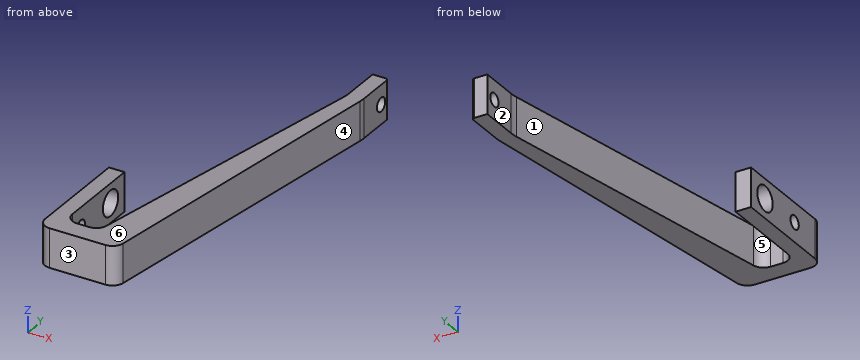
```python
from build123d import *

# Parameters (mm, degrees)
F0_W     = 4
F0_H     = 25
F1_DEPTH = 10
F2_R     = 3
F3_R     = 10
F4_R     = 1.75
F5_DEPTH = 5
F6_R     = 3.25
F6_R_2   = 1.75
F7_DEPTH = 6
F8_R     = 0.7


# Not quite as in the source:
# - a feature names something its author has since deleted; it is built from what else it names


with BuildPart() as f1:
    # F0 (on Top) → F1 (new body)
    with BuildSketch(Plane.XY):
        with Locations((2, 17.5)):
            Rectangle(F0_W, F0_H)
        Polygon((0, 5), (0, 0), (20, 0), (31.84, 84.7), (31.84, 95.7), (27.84, 95.7), (27.84, 84.7), (12.6761412248, 5), (4, 5), align=None)
    extrude(amount=F1_DEPTH)

    # F2
    f2_edges = [f1.edges().sort_by_distance(p)[0] for p in [
        (12.676141, 5, 5),
        (4, 5, 5),
        (0, 0, 5),
        (20, 0, 5),
    ]]
    fillet(f2_edges, radius=F2_R)

    # F3
    f3_edges = [f1.edges().sort_by_distance(p)[0] for p in [
        (27.84, 84.7, 5),
        (31.84, 84.7, 5),
    ]]
    fillet(f3_edges, radius=F3_R)

    # F4 (on face) → F5 (cut)
    with BuildSketch(Plane.YZ.offset(31.84)):
        with Locations((92.7, 5)):
            Circle(F4_R)
    extrude(amount=-F5_DEPTH, mode=Mode.SUBTRACT)

    # F6 (on face) → F7 (cut)
    with BuildSketch(Plane(origin=(0, 0, 0), x_dir=(0, -1, 0), z_dir=(-1, 0, 0))):
        with Locations((-24.1, 5)):
            Circle(F6_R)
        with Locations((-11.6, 5)):
            Circle(F6_R_2)
    extrude(amount=-F7_DEPTH, mode=Mode.SUBTRACT)

    # F8
    f8_edges = [f1.edges().sort_by_distance(p)[0] for p in [
        (31.84, 95.7, 5),
    ]]
    fillet(f8_edges, radius=F8_R)


solid = f1.part
```
Part model, mm, in its own coordinate system. Face numbers are marked on the shaded views. A direction names the side the tool comes from. Round coordinates to 2 decimals unless told otherwise and drop trailing zeros. Write each loop counter-clockwise with the first axis right and the second up, starting at its lowest first coordinate (ties: lowest second). Pieces come first, ordered by that corner, then holes.
Item 1: Cut at D-D, the plane x = 23. Give the cut face in (y, z).
Results:
outline: (21.46, 0) - (59.26, 0) - (59.26, 10) - (21.46, 10) - close
Item 2: Cut at C-C, the plane y = 11.6. Give the cut face in (x, z).
Results:
outline: (0, 0) - (4, 0) - (4, 3.25) - (0, 3.25) - close; (0, 6.75) - (4, 6.75) - (4, 10) - (0, 10) - close; (13.93, 0) - (21.62, 0) - (21.62, 10) - (13.93, 10) - close
Item 3: Probe L1, parallel to Z at x = 1.9, y = 24.1; L2, parallel to Z at x = 0.95, y = 11.6; L3, parallel to X at y = 10, z = 3.75. List the from-to ranges inside material, lowest first.
Results:
L1: z = 0 to 1.75, 8.25 to 10
L2: z = 0 to 3.25, 6.75 to 10
L3: x = 0 to 4, 13.63 to 21.4
Item 4: Two-plate mould, pull along X, no slides. Class the marked faces 4, 5 and 6: +X half, -X half, draft (parallel to the pull), parting line (faces both ways), or undercut.
Results:
face 4: +X half
face 5: undercut
face 6: draft
Item 5: Which spindle directions (+Z, -Z, +X, -X, +Y, -Y) get a long thin tool onto all of the face, cutting with end or side? Do the marked faces 1, 2 and 3. Say none if no direction does.
Results:
face 1: +Z, -Z, +Y
face 2: +Z, -Z, -X, +Y
face 3: +Z, -Z, +X, -X, -Y
Item 6: Cut at B-B, the plane z = 5. Count the separate pieces of the cut face and the enclosed holes in it, plus the area to 3 significant figures.
Results:
separate pieces: 4
enclosed holes: 0
area: 671 mm2
Item 7: Drop flat-ended pins along their axis: pin 1 Ø1 at (x, z) = (8, 3.5) entering from +Y; pin 2 Ø2 at (x, z) = (3, 6.5) entering from +Y; pin 3 Ø6 at (x, z) = (9, 2) entering from +Y. Give the stop position or say it passes through.
Results:
pin 1: stops at y = 5
pin 2: stops at y = 30
pin 3: stops at y = 5.61
Item 8: Cut at A-A, the plane y = 92.7. Give the cut face in (x, z).
Results:
outline: (27.84, 0) - (31.84, 0) - (31.84, 3.25) - (27.84, 3.25) - close; (27.84, 6.75) - (31.84, 6.75) - (31.84, 10) - (27.84, 10) - close
